Autodesk Inventor part; units mm, degrees
ref_plane "YZ Plane" through (0, 0, 0) normal (1, 0, 0) x (0, 1, 0)
ref_plane "XZ Plane" through (0, 0, 0) normal (0, 1, 0) x (-1, 0, 0)
ref_plane "XY Plane" through (0, 0, 0) normal (0, 0, 1) x (1, 0, 0)
sketch "Sketch1" plane through (0, 0, 0) normal (1, 0, 0) x (0, 1, 0)
  line L0 (0, 13.93) -> (0, -13.93) construction
  line L1 (-6.93, 0) -> (6.93, 0) construction
  line L2 (4.95, 9.95) -> (-4.95, 9.95)
  line L3 (-4.95, 9.95) -> (-4.95, -9.95)
  line L4 (-4.95, -9.95) -> (4.95, -9.95)
  line L5 (4.95, -9.95) -> (4.95, 9.95)
  point P0 (0, 0)
  dimension "d0" = 9.9
  dimension "d1" = 19.9
extrude "Extrusion1" add sketch "Sketch1" along normal blind 2
sketch "Sketch2" plane through (2, 0, 0) normal (1, 0, 0) x (0, 0, -1)
  circle A0 centre (0, 0) radius 1.65
  dimension "d4" = 3.3
extrude "Extrusion2" add sketch "Sketch2" along normal blind 3
fillet "Fillet1" radius 0.5 2 edges at (2, 0, 1.65) (5, 0, 1.65)
fillet "Fillet2" radius 0.5 12 edges at (2, -4.95, 0) (2, 0, 9.95) (1, -4.95, 9.95) (0, -4.95, 0) (1, -4.95, -9.95) (2, 0, -9.95) (0, 0, -9.95) (1, 4.95, -9.95) (0, 4.95, 0) (2, 4.95, 0) (1, 4.95, 9.95) (0, 0, 9.95)
properties part number "10x20-sample-bottom-V1"
Part model, mm, in its own coordinate system. A direction names the side the tool comes from. Round coordinates to 2 decimals unless told otherwise and drop trailing zeros. Order: outer loops, then holes, each group sorted by start corner. A loop starts at its lowest first (then second) coordinate and runs counter-clockwise, first axis right, second up. Notation, with made-up numbers: M -6.75,87 L 13.25,87 A12 cw 13.25,105 Z; hole C 37,46.5 d1. An arc over 180 degrees is marked long. Put each result on its own line as item: value. Start each with the question number.
1. Slice it at B-B on z = 2.5. List the corners of the cut face in (x, y).
2. Slice it at C-C on x = 4.05. List the corners of the cut face in (y, z).
3. Drill centre lines: probe 1 along X at (y, z) = (-1, 3.5); probe 2 along Z at (x, y) = (4.5, 1); probe 3 along Y at (x, z) = (2.5, -1.25). Where is each one in solid material? Low to high. Write a range as [from, to].
4. Tool access for faces 1 (the face through (3.486, -1.115, 1.216)), 2 (the face through (1, 0, 9.95)): list every direction of +Z, -Z, +X, -X, +Y, -Y with a clear straight run to the whole face (end or side of a thin tool).
5. Slice it at A-A on y = 0. List the corners of the cut face in (x, z).
6. Slice it at D-D on y = 3. List the corners of the cut face in (x, z), then the cut area to 3 significant figures.
Findings:
1. outline: M 0,-4.45 A0.5 ccw 0.5,-4.95 L 1.5,-4.95 A0.5 ccw 2,-4.45 L 2,4.45 A0.5 ccw 1.5,4.95 L 0.5,4.95 A0.5 ccw 0,4.45 Z
2. outline: C 0,0 d3.3
3. probe 1: [0, 2]
3. probe 2: [-1.31, 1.31]
3. probe 3: [-1.08, 1.08]
4. face 1: +X
4. face 2: +Z, +X, -X, +Y, -Y
5. outline: M 0,-9.45 A0.5 ccw 0.5,-9.95 L 1.5,-9.95 A0.5 ccw 2,-9.45 L 2,-2.15 A0.5 cw 2.5,-1.65 L 4.5,-1.65 A0.5 ccw 5,-1.15 L 5,1.15 A0.5 ccw 4.5,1.65 L 2.5,1.65 A0.5 cw 2,2.15 L 2,9.45 A0.5 ccw 1.5,9.95 L 0.5,9.95 A0.5 ccw 0,9.45 Z
6. outline: M 0,-9.45 A0.5 ccw 0.5,-9.95 L 1.5,-9.95 A0.5 ccw 2,-9.45 L 2,9.45 A0.5 ccw 1.5,9.95 L 0.5,9.95 A0.5 ccw 0,9.45 Z
6. area: 39.6 mm2
